```python
from build123d import *

# Parameters (mm, degrees)
F1_DEPTH = 27.2
F2_D     = 3
F3_D     = 3
F4_ANGLE = 180


with BuildPart() as f1:
    # F0 (on Front) → F1 (new body)
    with BuildSketch(Plane.XZ):
        with BuildLine():
            ThreePointArc((-44.7051230669, 7.7739851549), (-41.2051230669, 4.2739851549), (-37.7051230669, 7.7739851549))
            ThreePointArc((-37.7051230669, 7.7739851549), (-41.2051230669, 11.2739851549), (-44.7051230669, 7.7739851549))
        make_face()
        with BuildLine():
            ThreePointArc((-44.7051230669, 7.7739851549), (-41.2051230669, 11.2739851549), (-37.7051230669, 7.7739851549))
            Line((-37.7051230669, 7.7739851549), (-37.7051230669, 13.2739851549))
            Line((-37.7051230669, 13.2739851549), (-44.7051230669, 13.2739851549))
            Line((-44.7051230669, 13.2739851549), (-44.7051230669, 7.7739851549))
        make_face()
        with BuildLine():
            Line((-44.7051230669, 13.2739851549), (-37.7051230669, 13.2739851549))
            Line((-37.7051230669, 13.2739851549), (-22.2314571059, 13.2739851549))
            ThreePointArc((-22.2314571059, 13.2739851549), (-25.7032370007, 16.3304264081), (-23.1114218713, 20.1615598053))
            Line((-23.1114218713, 20.1615598053), (-69.2051230669, 20.1615598053))
            ThreePointArc((-69.2051230669, 20.1615598053), (-70.6193366293, 19.5757733676), (-71.2051230669, 18.1615598053))
            Line((-71.2051230669, 18.1615598053), (-71.2051230669, 15.2739851549))
            ThreePointArc((-71.2051230669, 15.2739851549), (-70.6193366293, 13.8597715926), (-69.2051230669, 13.2739851549))
            Line((-69.2051230669, 13.2739851549), (-44.7051230669, 13.2739851549))
        make_face()
        with BuildLine():
            Line((-22.2314571059, 20.1615598053), (-22.2314571059, 13.2739851549))
            ThreePointArc((-22.2314571059, 13.2739851549), (-19.7565833717, 14.2991114208), (-18.7314571059, 16.7739851549))
            ThreePointArc((-18.7314571059, 16.7739851549), (-20.0901813972, 19.5425476591), (-23.1114218713, 20.1615598053))
            Line((-23.1114218713, 20.1615598053), (-22.2314571059, 20.1615598053))
        make_face()
        with BuildLine():
            ThreePointArc((-23.1114218713, 20.1615598053), (-25.7032370007, 16.3304264081), (-22.2314571059, 13.2739851549))
            Line((-22.2314571059, 13.2739851549), (-22.2314571059, 20.1615598053))
            Line((-22.2314571059, 20.1615598053), (-23.1114218713, 20.1615598053))
        make_face()
    extrude(amount=-F1_DEPTH)

    # F2 (through all)
    with Locations(Plane.XZ):
        with Locations((-41.2051230669, 7.7739851549)):
            Hole(F2_D / 2)

    # F3 (through all)
    with Locations(Plane.XZ):
        with Locations((-22.2314571059, 16.7739851549)):
            Hole(F3_D / 2)


with BuildPart() as f1_1:
    # F4: moved
    add(f1.part.rotate(Axis((-46.1582724691, 0, 20.1615598053), (-1, 0, 0)), F4_ANGLE))


solid = f1_1.part
```
Could you check a few things on this model? Use its own coordinates, in mm. A direction names the side the tool comes from. Coordinates: 2 decimals unless noted, no trailing zeros. Write each loop counter-clockwise with the first axis right and the second up, starting at its lowest first coordinate (ties: lowest second). Pieces come first, ordered by that corner, then holes. Notation, with made-up numbers: (81.25, -10.75) -> (96.25, -10.75) arc R36 ccw to (96.25, 23.25) -> close; hole circle Ø3 at (42.5, 40). An arc over 180 degrees is marked (long way). Write item = value, one per line. Start each with the question number.
(1) We'd pull the mould along X, two halves only. Please class faces 6 (the face through (-40.015, -13.79, 33.462)), 7 (the face through (-57, -13, 27.049)), 8 (the face through (-70.63, -13.41, 26.45)): released by +X, released by -X, zero draft, split by the parting line, or undercut.
(2) I want a section at C-C (x = -52). Please give me the cut outline in (y, z).
(3) Will these pins go through, and if not, where does the flat tip stop? pin 1 (13.5 mm diameter, centred on x = -39.5, y = -20.5, fed in from -Z); pin 2 (4 mm diameter, centred on x = -61, z = 31, fed in from -Y); pin 3 (6 mm diameter, centred on y = -20, z = 28.5, fed in from +X); pin 4 (12.5 mm diameter, centred on x = -28.5, y = -9, fed in from +Z).
(4) Which directions (+Z, -Z, +X, -X, +Y, -Y) give clear straight access to the entire face, cutting with the end or side of a thin tool? Please do faces 1 (the face through (-21.906, -13.79, 25.013)), 2 (the face through (-44.705, -13, 30)), 3 (the face through (-46, -13, 20.162)), 4 (the face through (-41.28, -13.41, 36.05)), 5 (the face through (-30, -13, 27.049)).
(5) I need wall thicknesses on line 1 (X direction, y = -23, z = 23.5); line 2 (Z direction, x = -42, y = -22.5); line 3 (Z direction, x = -60, y = -20). Which ranges of each line are inside material? Lowest first, please. Write a range as [from, to].
(6) I want a section at A-A (y = -15.75). Please give me the cut outline in (x, z).
(7) I want a section at B-B (z = 28). Please give me the cut outline in (x, y).
Result set:
q1.face_6 = undercut
q1.face_7 = zero draft
q1.face_8 = released by -X
q2.outline = (-27.2, 20.16) -> (0, 20.16) -> (0, 27.05) -> (-27.2, 27.05) -> close
q3.pin_1 = 20.16
q3.pin_2 = through
q3.pin_3 = -19.33
q3.pin_4 = 27.05
q4.face_1 = +Y, -Y
q4.face_2 = +Z, -X, +Y, -Y
q4.face_3 = -Z, -X, +Y, -Y
q4.face_4 = +Z, +Y, -Y
q4.face_5 = +Z, +X, +Y, -Y
q5.line_1 = [-71.21, -23.73], [-20.73, -18.73]
q5.line_2 = [20.16, 31.28], [33.82, 35.96]
q5.line_3 = [20.16, 27.05]
q6.outline = (-71.21, 22.16) arc R2 ccw to (-69.21, 20.16) -> (-23.11, 20.16) arc R3.5 ccw (long way) to (-22.23, 27.05) -> (-37.71, 27.05) -> (-37.71, 32.55) arc R3.5 ccw to (-44.71, 32.55) -> (-44.71, 27.05) -> (-69.21, 27.05) arc R2 ccw to (-71.21, 25.05) -> close; hole circle Ø3 at (-41.21, 32.55); hole circle Ø3 at (-22.23, 23.55)
q7.outline = (-44.71, -27.2) -> (-37.71, -27.2) -> (-37.71, 0) -> (-44.71, 0) -> close
